from build123d import *

# Parameters (mm, degrees)
BOSS_EXTRUDE1_DEPTH = 6.35
SKETCH5_R           = 6.858
BOSS_EXTRUDE2_DEPTH = 11.938
BOSS_EXTRUDE2_TAPER = 1.783333333


with BuildPart() as part:
    # Sketch2 → Revolve1 (revolve)
    with BuildSketch(Plane(origin=(0, 0, 0), x_dir=(0, 0, -1), z_dir=(1, 0, 0)), mode=Mode.PRIVATE) as revolve1_sk:
        Polygon((-23.876, 0), (-6.35, 0), (-6.35, 9.0805), (-19.876, 9.0805), (-19.876, 8.5805), (-20.376, 8.5805), (-20.376, 9.0805), (-20.876, 9.0805), (-21.376, 8.5805), (-21.376, 5.3975), (-22.376, 5.3975), (-22.376, 7.3025), (-23.876, 7.3025), align=None)
    revolve(revolve1_sk.sketch.rotate(Axis((0, 0, 23.876), (0, 0, -1)), 90), axis=Axis((0, 0, 23.876), (0, 0, -1)))

    # Sketch3 → Boss-Extrude1 (add)
    with BuildSketch(Plane(origin=(0, 0, 6.35), x_dir=(-1, 0, 0), z_dir=(0, 0, -1))):
        Polygon((0, 11.91506618), (-10.31875, 5.95753309), (-10.31875, -5.95753309), (0, -11.91506618), (10.31875, -5.95753309), (10.31875, 5.95753309), align=None)
    extrude(amount=BOSS_EXTRUDE1_DEPTH)


with BuildPart() as body_2:
    # Sketch5 → Boss-Extrude2 (new body)
    with BuildSketch(Plane(origin=(0, 0, 0), x_dir=(-1, 0, 0), z_dir=(0, 0, -1))):
        Circle(SKETCH5_R)
    extrude(amount=BOSS_EXTRUDE2_DEPTH, taper=BOSS_EXTRUDE2_TAPER)


with BuildPart() as part_1:
    add(part.part)

    # Combine1: union body 2
    add(body_2.part)

    # Sketch9 → Cut-Revolve2 (revolve, cut)
    with BuildSketch(Plane(origin=(0, 0, 0), x_dir=(0, 0, -1), z_dir=(1, 0, 0)), mode=Mode.PRIVATE) as cut_revolve2_sk:
        Polygon((-23.876, 4.7625), (-1.905, 4.7625), (-1.905, 3.81), (-0.956760375, 3.81), (-0.468380864, 4.6228), (11.938, 4.6228), (11.938, 0), (-23.876, 0), align=None)
    revolve(cut_revolve2_sk.sketch.rotate(Axis((0, 0, -11.938), (0, 0, 1)), 90), axis=Axis((0, 0, -11.938), (0, 0, 1)), mode=Mode.SUBTRACT)


solid = part_1.part
Work out the finished part from the listing and answer in its coordinate system (mm). A direction names the side the tool comes from. Give positions to 0.01 mm unless a question says otherwise; leave off trailing zeros. Order: outer loops, then holes, each group sorted by start corner. A loop starts at its lowest first (then second) coordinate and runs counter-clockwise, first axis right, second up. Notation, with made-up numbers: (54.5, 62.25) -> (66.5, 62.25) arc R28 ccw to (66.5, 98.25) -> close; hole circle Ø1 at (60.25, 71). An arc over 180 degrees is marked (long way). Answer as a JSON object with one key per item and string values. Group by question number.
1. Section A-A on z = 11.5 is taken. Determine the outline of the cut face in (x, y) (1 decimal).
2. Section B-B on z = -6 is taken. Determine the outline of the cut face in (x, y), plus the area to 3 significant figures.
3. Consider line 1 along Y through (x, z) = (0, 8.5); line 2 along Y through (x, z) = (0, 1.75); line 3 along Z through (x, y) = (3.25, 10). Determine where each line is inside the solid, lowest interval first. Write a range as [from, to].
4. Flat-ended cylindrical pins translate along their axes: pin 1 Ø1 at (y, z) = (-6.5, 15.5) entering from -X; pin 2 Ø1.5 at (y, z) = (-0.5, 11) entering from -X; pin 3 Ø5 at (y, z) = (-8.5, 5.5) entering from +X. Find the tip coordinate at first contact, or state that the pin passes through.
5. The mould has two halves that part along Z. Classify faces 6 (the flat face through (5, 0, 23.876)), 7 (the flat face through (5.087, 8.978, 3.219)), 8 (the flat face through (6, 0, 21.376)): released by +Z, released by -Z, zero draft, split by the parting line, or undercut.
6. A tool of negligible diameter and unlimited length cuts with its end or side. For faces 1 (the flat face through (-5.087, -8.978, 3.219)), 2 (the cylindrical face through (-3.978, -3.648, 21.883)), 3 (the flat face through (-10.319, 0, 3)), 4 (the flat face through (-1, -4, 1.905)), 5 (the flat face through (5, -5, 0)), from which of +Z, -Z, +X, -X, +Y, -Y can it reach the whole face along a straight path? Write none if from no direction.
Result sheet:
{
 "1": {"outline": "circle Ø18.2 at (0, 0); hole circle Ø9.5 at (0, 0)"},
 "2": {"outline": "circle Ø13.34 at (0, 0); hole circle Ø9.25 at (0, 0)", "area": "72.7 mm^2"},
 "3": {"line 1": "y = [-9.08, -4.76], [4.76, 9.08]", "line 2": "y = [-11.92, -3.81], [3.81, 11.92]", "line 3": "z = [0, 6.35]"},
 "4": {"pin 1": "stops at x = -6.82", "pin 2": "stops at x = -9.08", "pin 3": "stops at x = 10.25"},
 "5": {"face 6": "released by +Z", "face 7": "zero draft", "face 8": "undercut"},
 "6": {"face 1": "+Z, -Z, -X, -Y", "face 2": "none", "face 3": "+Z, -Z, -X, +Y, -Y", "face 4": "+Z", "face 5": "-Z"}
}
